from build123d import *

# Parameters (mm, degrees)
SKETCH1_W               = 300
SKETCH1_H               = 400
BOSS_EXTRUDE1_DEPTH     = 5
CUT_EXTRUDE2_DEPTH      = 400
CUT_EXTRUDE3_DEPTH      = 251.049995001
CUT_EXTRUDE3_DEPTH_BACK = 251.049995001
SKETCH7_W               = 2
SKETCH7_H               = 100
SKETCH8_W               = 284
SKETCH8_H               = 395
CUT_EXTRUDE4_DEPTH      = 2.5
FILLET1_R               = 10
CUT_EXTRUDE5_DEPTH      = 251.049995001
CUT_EXTRUDE5_DEPTH_BACK = 251.049995001


with BuildPart() as part:
    # Sketch1 → Boss-Extrude1 (new body)
    with BuildSketch(Plane(origin=(0, 0, 0), x_dir=(1, 0, 0), z_dir=(0, 1, 0))):
        Rectangle(SKETCH1_W, SKETCH1_H)
    extrude(amount=BOSS_EXTRUDE1_DEPTH)

    # Sketch6 → Cut-Extrude2 (cut)
    with BuildSketch(Plane.XY.offset(200)):
        with BuildLine():
            Line((145, 0), (150, 0))
            Line((150, 0), (150, 5))
            ThreePointArc((150, 5), (148.535533906, 1.464466094), (145, 0))
        make_face()
    extrude(amount=-CUT_EXTRUDE2_DEPTH, mode=Mode.SUBTRACT)

    # Sketch7 → Cut-Extrude3 (cut, two sides: drawn at the far end of the back side and taken through both)
    with BuildSketch(Plane(origin=(0, 5, 0), x_dir=(1, 0, 0), z_dir=(0, 1, 0)).offset(-CUT_EXTRUDE3_DEPTH_BACK)):
        with Locations((142.5, 0)):
            Rectangle(SKETCH7_W, SKETCH7_H)
        with Locations((142.5, 133.333333333)):
            Rectangle(SKETCH7_W, SKETCH7_H)
        with Locations((142.5, -133.333333333)):
            Rectangle(SKETCH7_W, SKETCH7_H)
    extrude(amount=CUT_EXTRUDE3_DEPTH + CUT_EXTRUDE3_DEPTH_BACK, mode=Mode.SUBTRACT)

    # Sketch8 → Cut-Extrude4 (cut)
    with BuildSketch(Plane(origin=(0, 5, 0), x_dir=(1, 0, 0), z_dir=(0, 1, 0))):
        with Locations((-5.5, 0)):
            Rectangle(SKETCH8_W, SKETCH8_H)
    extrude(amount=-CUT_EXTRUDE4_DEPTH, mode=Mode.SUBTRACT)

    # Fillet1
    fillet1_edges = [part.edges().sort_by_distance(p)[0] for p in [
        (-150, 2.5, 200),
        (-150, 2.5, -200),
        (136.5, 3.75, -197.5),
        (136.5, 3.75, 197.5),
        (-147.5, 3.75, 197.5),
        (-147.5, 3.75, -197.5),
    ]]
    fillet(fillet1_edges, radius=FILLET1_R)

    # Sketch9 → Cut-Extrude5 (cut, two sides: drawn at the far end of the back side and taken through both)
    with BuildSketch(Plane(origin=(0, 5, 0), x_dir=(1, 0, 0), z_dir=(0, 1, 0)).offset(-CUT_EXTRUDE5_DEPTH_BACK)):
        with BuildLine():
            Line((140, 200), (150, 200))
            Line((150, 200), (150, 190))
            ThreePointArc((150, 190), (147.071067812, 197.071067812), (140, 200))
        make_face()
        with BuildLine():
            Line((150, -200), (150, -190))
            ThreePointArc((150, -190), (147.071067812, -197.071067812), (140, -200))
            Line((140, -200), (150, -200))
        make_face()
    extrude(amount=CUT_EXTRUDE5_DEPTH + CUT_EXTRUDE5_DEPTH_BACK, mode=Mode.SUBTRACT)


solid = part.part
Can you work these out from the model? Positions are in its coordinate system, mm. A direction names the side the tool comes from. Give positions to 0.01 mm unless a question says otherwise; leave off trailing zeros. Order: outer loops, then holes, each group sorted by start corner. A loop starts at its lowest first (then second) coordinate and runs counter-clockwise, first axis right, second up. Notation, with made-up numbers: M 13,-17 L 69,-17 A22 cw 69,-8 Z; hole C 72.25,28 d8. An arc over 180 degrees is marked long. Use one line per item in the form item = value. Start each with the question number.
Item 1: We'd pull the mould along Z, two halves only. Please class faces 3 (the cylindrical face through (-147.15, 2.54, -196.99)), 4 (the cylindrical face through (-147.15, 2.54, 196.99)), 5 (the cylindrical face through (133.65, 3.73, -194.49)): +Z half, -Z half, draft (parallel to the pull), parting line (faces both ways), or undercut.
Item 2: If we section it at B-B (x = -15): Write out the boundary of the cut face in (y, z).
Item 3: If we section it at D-D (z = -78): Write out the boundary of the cut face in (x, y), then the cut area to 3 significant figures.
Item 4: If we section it at A-A (z = 12.5): Write out the boundary of the cut face in (x, y).
Item 5: If we section it at C-C (y = 3.55): Write out the boundary of the cut face in (x, z), then the cut area to 3 significant figures.
Item 6: If I drill on line 1 along X through (y, z) = (4.3, 130); line 2 along Z through (x, y) = (-1, 4.5); line 3 along X through (y, z) = (2.6, -117.5), over which ranges is the centre line in solid material (lowest first)?
Item 7: For faces 1 (the flat face through (-5, 0, -3)), 2 (the cylindrical face through (-144.49, 3.73, 194.65)), which set-ups out of +Z, -Z, +X, -X, +Y, -Y let a thin tool reach every point of the face, with its end or its side?
Item 8: Will these pins go through, and if not, where does the flat tip stop? pin 1 Ø2 at (x, y) = (142.5, 2.5) entering from -Z; pin 2 Ø0.6 at (x, y) = (142.5, 2) entering from +Z (3 decimals); pin 3 Ø1 at (y, z) = (0.5, 60) entering from +X; pin 4 Ø2 at (x, z) = (42, -27) entering from -Y.
Outcome:
q1.face_3 = -Z half
q1.face_4 = +Z half
q1.face_5 = undercut
q2.outline = M 0,-200 L 5,-200 L 5,-197.5 L 2.5,-197.5 L 2.5,197.5 L 5,197.5 L 5,200 L 0,200 Z
q3.outline = M -150,0 L 145,0 A5 ccw 150,5 L 136.5,5 L 136.5,2.5 L -147.5,2.5 L -147.5,5 L -150,5 Z
q3.area = 785 mm2
q4.outline = M -150,0 L 141.5,0 L 141.5,5 L 136.5,5 L 136.5,2.5 L -147.5,2.5 L -147.5,5 L -150,5 Z; M 143.5,0 L 145,0 A5 ccw 150,5 L 143.5,5 Z
q5.outline = M -150,-190 A10 ccw -140,-200 L 140,-200 A10 ccw 149.79,-192.06 L 149.79,192.06 A10 ccw 140,200 L -140,200 A10 ccw -150,190 Z; hole M -147.5,-187.5 A10 ccw -137.5,-197.5 L 126.5,-197.5 A10 ccw 136.5,-187.5 L 136.5,187.5 A10 ccw 126.5,197.5 L -137.5,197.5 A10 ccw -147.5,187.5 Z; hole M 141.5,-183.33 L 143.5,-183.33 L 143.5,-83.33 L 141.5,-83.33 Z; hole M 141.5,-50 L 143.5,-50 L 143.5,50 L 141.5,50 Z; hole M 141.5,83.33 L 143.5,83.33 L 143.5,183.33 L 141.5,183.33 Z
q5.area = 7,140 mm2
q6.line_1 = -150 to -147.5, 136.5 to 141.5, 143.5 to 149.95
q6.line_2 = -200 to -197.5, 197.5 to 200
q6.line_3 = -150 to -147.5, 136.5 to 141.5, 143.5 to 149.39
q7.face_1 = +Z, -Z, +X, -X, -Y
q7.face_2 = +Y
q8.pin_1 = -199.89
q8.pin_2 = 199.755
q8.pin_3 = 148
q8.pin_4 = 0
